Work out the finished part from the listing and answer in its coordinate system (mm). A direction names the side the tool comes from. Give positions to 0.01 mm unless a question says otherwise; leave off trailing zeros. Loops run counter-clockwise (first coordinate to the right, second up) from the corner with the lowest first, then second, coordinate; pieces in that order, holes last. Notation, with made-up numbers: (-13.75, 87.5) - (43.25, 87.5) arc R3 ccw to (43.25, 92.5) - close; hole circle Ø2 at (35.5, -39). An arc over 180 degrees is marked (long way). One line per item, written item: value.
from build123d import *

# Parameters (mm, degrees)
BOSS_EXTRUDE1_DEPTH        = 5
BOSS_EXTRUDE2_DEPTH        = 5
F_3_2_3_2_DIAMETER_HOLE1_D = 3.2


with BuildPart() as part:
    # Sketch1 → Boss-Extrude1 (new body)
    with BuildSketch(Plane(origin=(0, 0, 0), x_dir=(1, 0, 0), z_dir=(0, 1, 0))):
        with BuildLine():
            Line((-196.961550602, 34.729635533), (-187.113473072, 32.993153757))
            ThreePointArc((-187.113473072, 32.993153757), (-190, 0), (-187.113473072, -32.993153757))
            Line((-187.113473072, -32.993153757), (-196.961550602, -34.729635533))
            ThreePointArc((-196.961550602, -34.729635533), (-200, 0), (-196.961550602, 34.729635533))
        make_face()
    extrude(amount=BOSS_EXTRUDE1_DEPTH)

    # Sketch9 → Boss-Extrude2 (add)
    with BuildSketch(Plane(origin=(0, 5, 0), x_dir=(1, 0, 0), z_dir=(0, 1, 0))):
        with BuildLine():
            Line((-199.749843554, 10), (-189.73665961, 10))
            ThreePointArc((-189.73665961, 10), (-190, 0), (-189.73665961, -10))
            Line((-189.73665961, -10), (-199.749843554, -10))
            ThreePointArc((-199.749843554, -10), (-200, 0), (-199.749843554, 10))
        make_face()
    extrude(amount=BOSS_EXTRUDE2_DEPTH)

    # Ø3.2 (3.2) Diameter Hole1 (through all)
    with Locations(Plane(origin=(0, 5, 0), x_dir=(1, 0, 0), z_dir=(0, 1, 0))):
        with Locations((-194.257966128, 16.995369836), (-193.331747968, 25.452607483), (-194.257966128, -16.995369836), (-193.331747968, -25.452607483)):
            Hole(F_3_2_3_2_DIAMETER_HOLE1_D / 2)


solid = part.part
1. Section D-D (y = 9) is taken. Write down the section's boundary in (x, z), and give its area (3 significant figures).
Output:
outline: (-199.75, -10) - (-189.74, -10) arc R190 cw to (-189.74, 10) - (-199.75, 10) arc R200 ccw to start
area: 200 mm²
2. Flat-ended cylindrical pins translate along their axes: pin 1 Ø2.5 at (x, y) = (-195, 6.5) entering from +Z; pin 2 Ø5 at (x, z) = (-192, 22) entering from +Y; pin 3 Ø3 at (x, y) = (-194, 2.5) entering from +Z; pin 4 Ø1.9 at (x, z) = (-193.33, 25.45) entering from -Y. Find the tip coordinate at first contact, or state that the pin passes through.
Output:
pin 1: stops at z = 10
pin 2: stops at y = 5
pin 3: stops at z = 34.47
pin 4: passes through
3. For faces 1 (the flat face through (-192.106, 2.465, -33.874)), 2 (the flat face through (-193, 5, 22)), 3 (the flat face through (-195, 7, -10)), determine the directions among +Z, -Z, +X, -X, +Y, -Y from which every point of the face is accessible in a straight line to the end or side of a thin tool.
Output:
face 1: -Z, +X, +Y, -Y
face 2: +Z, +X, -X, +Y
face 3: -Z, +X, -X, +Y
4. Find the intervals of material crossed by line 1 along Z through (x, y) = (-195.5, 2.75); line 2 along Z through (x, y) = (-193.25, 3.25); line 3 along Y through (x, z) = (-188.5, 27), in increasing order.
Output:
line 1: z = -34.47 to -18, -15.99 to 15.99, 18 to 34.47
line 2: z = -34.08 to -27.05, -23.85 to -18.24, -15.75 to 15.75, 18.24 to 23.85, 27.05 to 34.08
line 3: y = 0 to 5
5. Section B-B (y = 4) is taken. Write down the section's boundary in (x, z), and give its area (3 significant figures).
Output:
outline: (-196.96, -34.73) - (-187.11, -32.99) arc R190 cw to (-187.11, 32.99) - (-196.96, 34.73) arc R200 ccw to start; hole circle Ø3.2 at (-194.26, -17); hole circle Ø3.2 at (-194.26, 17); hole circle Ø3.2 at (-193.33, -25.45); hole circle Ø3.2 at (-193.33, 25.45)
area: 649 mm²
6. The mould has two halves that part along X. Classify faces 4 (the flat face through (-191.97, 2.46, 33.85)), 5 (the flat face through (-193, 5, -23)), 6 (the cylindrical face through (-194.81, 2.47, 26.07)): released by +X, released by -X, zero draft, split by the parting line, or undercut.
Output:
face 4: released by +X
face 5: zero draft
face 6: undercut
7. Section C-C (x = -198.25) is taken. Write down the section's boundary in (y, z).
Output:
outline: (0, -26.4) - (5, -26.4) - (5, -10) - (10, -10) - (10, 10) - (5, 10) - (5, 26.4) - (0, 26.4) - close
8. Section A-A (z = -16) is taken. Write down the section's boundary in (x, y), and give its area (3 significant figures).
Output:
outline: (-199.36, 0) - (-195.51, 0) - (-195.51, 5) - (-199.36, 5) - close; (-193.01, 0) - (-189.33, 0) - (-189.33, 5) - (-193.01, 5) - close
area: 37.6 mm²
